Build history of the part. All positions in model axes, mm. Round coordinates to 2 decimals unless told otherwise and drop trailing zeros. Write each loop counter-clockwise with the first axis right and the second up, starting at its lowest first coordinate (ties: lowest second). Pieces come first, ordered by that corner, then holes. Notation, with made-up numbers: (37.5, 42) -> (79.5, 42) arc R6 ccw to (79.5, 53) -> close; hole circle Ø1 at (87.5, 27). An arc over 180 degrees is marked (long way). One line per question, with ' | ' between items.
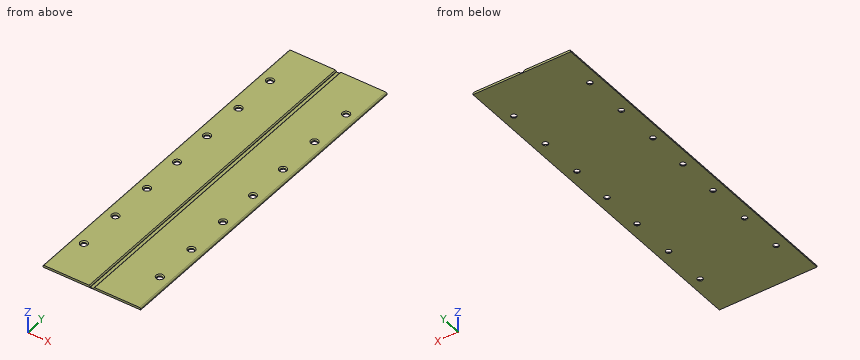
from build123d import *

# Parameters (mm, degrees)
ESQUISSE1_W             = 90
ESQUISSE1_H             = 320
BOSS_EXTRU_1_DEPTH      = 2
ESQUISSE2_R             = 2.5
ENL_V_MAT_EXTRU_1_DEPTH = 45
CONG_2_R                = 1
CHANFREIN1_SIZE         = 1
ENL_V_START             = 2
ESQUISSE3_W             = 3
ESQUISSE3_H             = 320
ENL_V_MAT_EXTRU_2_DEPTH = 1.5
CHANFREIN2_SIZE         = 1


with BuildPart() as part:
    # Esquisse1 → Boss.-Extru.1 (new body)
    with BuildSketch(Plane.XY):
        Rectangle(ESQUISSE1_W, ESQUISSE1_H)
    extrude(amount=BOSS_EXTRU_1_DEPTH)

    # Esquisse2 → Enlèv. mat.-Extru.1 (cut)
    with BuildSketch(Plane.XY.offset(2)):
        with Locations((-35, 120.982014683)):
            Circle(ESQUISSE2_R)
        with Locations((35, 120.982014683)):
            Circle(ESQUISSE2_R)
        with Locations((35, 80)):
            Circle(ESQUISSE2_R)
        with Locations((-35, 80)):
            Circle(ESQUISSE2_R)
        with Locations((-35, 39.017985317)):
            Circle(ESQUISSE2_R)
        with Locations((35, 39.017985317)):
            Circle(ESQUISSE2_R)
        with Locations((35, 0)):
            Circle(ESQUISSE2_R)
        with Locations((-35, 0)):
            Circle(ESQUISSE2_R)
        with Locations((-35, -39.017985317)):
            Circle(ESQUISSE2_R)
        with Locations((35, -39.017985317)):
            Circle(ESQUISSE2_R)
        with Locations((35, -80)):
            Circle(ESQUISSE2_R)
        with Locations((-35, -80)):
            Circle(ESQUISSE2_R)
        with Locations((35, -120.982014683)):
            Circle(ESQUISSE2_R)
        with Locations((-35, -120.982014683)):
            Circle(ESQUISSE2_R)
    extrude(amount=-ENL_V_MAT_EXTRU_1_DEPTH, mode=Mode.SUBTRACT)

    # Congé2
    cong_2_edges = [part.edges().sort_by_distance(p)[0] for p in [
        (45, 0, 2),
        (-45, 0, 2),
    ]]
    fillet(cong_2_edges, radius=CONG_2_R)

    # Chanfrein1
    chanfrein1_edges = [part.edges().sort_by_distance(p)[0] for p in [
        (-37.5, -39.017985317, 2),
        (-37.5, 0, 2),
        (32.5, 0, 2),
        (32.5, 39.017985317, 2),
        (-37.5, 39.017985317, 2),
        (-37.5, 80, 2),
        (32.5, 80, 2),
        (32.5, 120.982014683, 2),
        (-37.5, -120.982014683, 2),
        (32.5, -39.017985317, 2),
        (32.5, -80, 2),
        (-37.5, -80, 2),
        (32.5, -120.982014683, 2),
        (-37.5, 120.982014683, 2),
    ]]
    chamfer(chanfrein1_edges, length=CHANFREIN1_SIZE)

    # Esquisse3 → Enlèv. mat.-Extru.2 (cut)
    with BuildSketch(Plane.XY.offset(ENL_V_START)):
        Rectangle(ESQUISSE3_W, ESQUISSE3_H)
    extrude(amount=-ENL_V_MAT_EXTRU_2_DEPTH, mode=Mode.SUBTRACT)

    # Chanfrein2
    chanfrein2_edges = [part.edges().sort_by_distance(p)[0] for p in [
        (-1.5, 0, 2),
        (1.5, 0, 2),
    ]]
    chamfer(chanfrein2_edges, length=CHANFREIN2_SIZE)


solid = part.part
(1) Drop flat-ended pins along their axis: pin 1 (4.5 mm diameter, centred on x = 35, y = 120.98, fed in from +Z); pin 2 (0.9 mm diameter, centred on x = -0.5, y = 30.5, fed in from +Z); pin 3 (6 mm diameter, centred on x = -35, y = -120.98, fed in from +Z). Give the stop position or say it passes through.
Calculated:
pin 1: through | pin 2: z = 0.5 | pin 3: z = 1.5
(2) Slice it at A-A (y = -111). Write the cut outline in (x, z).
Calculated:
outline: (-45, 0) -> (45, 0) -> (45, 1) arc R1 ccw to (44, 2) -> (2.5, 2) -> (1.5, 1) -> (1.5, 0.5) -> (-1.5, 0.5) -> (-1.5, 1) -> (-2.5, 2) -> (-44, 2) arc R1 ccw to (-45, 1) -> close
(3) Wall check: line 1 (X direction, y = 48, z = 0.55); line 2 (X direction, y = 101.5, z = 1.7). Give the ranges that are in metal, low to high. Write a range as from..to.
Calculated:
line 1: -45..-1.5, 1.5..45 | line 2: -44.71..-2.2, 2.2..44.71
